Can you work these out from the model? Positions are in its coordinate system, mm. A direction names the side the tool comes from. Give positions to 0.01 mm unless a question says otherwise; leave off trailing zeros. Write each loop counter-clockwise with the first axis right and the second up, starting at its lowest first coordinate (ties: lowest second). Pieces come first, ordered by that corner, then holes.
1. Suppose I cut it at B-B (y = -6.25). Please give me the cut outline in (x, z), and give its area (3 significant figures).
2. Suppose I cut it at A-A (x = 12.5). Please give me the cut outline in (y, z), and give its area (3 significant figures).
3. On a 3-axis mill with a long thin cutter (end or side, diameter ignored), from which of +Z, -Z, +X, -X, +Y, -Y can I reach the whole of each face in a straight line? I mean faces 4 (the flat face through (4.413, -5, -5)), 5 (the flat face through (-5.428, -5, -5)). Say none if no direction works.
4. I'm going to push a flat-ended pin straight in: pin 1 (3 mm diameter, centred on y = -2.5, z = -2.5, fed in from +X). Where does the tip first touch, or does it pass through?
5. Suppose I cut it at C-C (z = -6). Please give me the cut outline in (x, y).
6. If I drill on probe 1 along Z at (x, y) = (4.5, -7); probe 2 along X at (y, z) = (-1.25, -9.5); probe 3 along Y at (x, z) = (4, -4), over which ranges is the centre line in solid material (lowest first)?
7. Thinking about a two-plate mould opening in Z: for faces 1 (the flat face through (9, -5, -15.296)), 2 (the flat face through (2, -10, -5)), 3 (the flat face through (5, -5, 14.704)), which applies, pulls with the +Z half, pulls with the -Z half, needs draft (parallel to the pull), parting line crosses it, or undercut?
```python
from build123d import *

# Parameters (mm, degrees)
F1_DEPTH    = 10
F2_R        = 0.5
F3_R        = 0.5
F4_T1_DEPTH = 11.5


# Not quite as in the source:
# - a fillet or chamfer that OpenCascade refuses, or shapes differently, is made with other operations: its cross-section is extruded or revolved along the edge and cut away or added


with BuildPart() as f1:
    # F0 (on Front) → F1 (new body)
    with BuildSketch(Plane.XZ):
        Polygon((14.5721812431, 14.7042763403), (-5.4278187569, 14.7042763403), (-5.4278187569, -25.2957236597), (14.5721812431, -25.2957236597), (14.5721812431, -15.2957236597), (4.4125382692, -15.2957236597), (4.4125382692, 4.7042763403), (14.5721812431, 4.7042763403), align=None)
    extrude(amount=F1_DEPTH)

    # F2
    f2_edges = [f1.edges().sort_by_distance(p)[0] for p in [
        (14.572181, -10, 9.704276),
        (4.572181, -10, 14.704276),
        (-5.427819, -10, -5.295724),
        (4.572181, -10, -25.295724),
        (14.572181, -10, -20.295724),
        (9.49236, -10, -15.295724),
        (4.412538, -10, -5.295724),
        (9.49236, -10, 4.704276),
    ]]
    fillet(f2_edges, radius=F2_R)

    # F3
    f3_edges = [f1.edges().sort_by_distance(p)[0] for p in [
        (14.572181, 0, 9.704276),
        (4.572181, 0, 14.704276),
        (-5.427819, 0, -5.295724),
        (4.572181, 0, -25.295724),
        (14.572181, 0, -20.295724),
        (9.49236, 0, -15.295724),
        (4.412538, 0, -5.295724),
        (9.49236, 0, 4.704276),
    ]]
    fillet(f3_edges, radius=F3_R)

    # F4: fillet of radius 0.5 on 16 edges, made by hand

    # F4_s2 → F4_t1 (cut)
    with BuildSketch(Plane.XZ.offset(-0.75)):
        with BuildLine():
            ThreePointArc((14.0721812431, -25.2957236597), (14.4257346337, -25.1492770503), (14.5721812431, -24.7957236597))
            Line((14.5721812431, -24.7957236597), (14.5721812431, -25.2957236597))
            Line((14.5721812431, -25.2957236597), (14.0721812431, -25.2957236597))
        make_face()
        with BuildLine():
            ThreePointArc((14.0721812431, -15.2957236597), (14.4257346337, -15.4421702691), (14.5721812431, -15.7957236597))
            Line((14.5721812431, -15.7957236597), (14.5721812431, -15.2957236597))
            Line((14.5721812431, -15.2957236597), (14.0721812431, -15.2957236597))
        make_face()
        with BuildLine():
            ThreePointArc((-5.4278187569, -24.7957236597), (-5.2813721475, -25.1492770503), (-4.9278187569, -25.2957236597))
            Line((-4.9278187569, -25.2957236597), (-5.4278187569, -25.2957236597))
            Line((-5.4278187569, -25.2957236597), (-5.4278187569, -24.7957236597))
        make_face()
        with BuildLine():
            ThreePointArc((14.5721812431, 5.2042763403), (14.4257346337, 4.8507229497), (14.0721812431, 4.7042763403))
            Line((14.0721812431, 4.7042763403), (14.5721812431, 4.7042763403))
            Line((14.5721812431, 4.7042763403), (14.5721812431, 5.2042763403))
        make_face()
        with BuildLine():
            ThreePointArc((14.5721812431, 14.2042763403), (14.4257346337, 14.5578297309), (14.0721812431, 14.7042763403))
            Line((14.0721812431, 14.7042763403), (14.5721812431, 14.7042763403))
            Line((14.5721812431, 14.7042763403), (14.5721812431, 14.2042763403))
        make_face()
        with BuildLine():
            ThreePointArc((-4.9278187569, 14.7042763403), (-5.2813721475, 14.5578297309), (-5.4278187569, 14.2042763403))
            Line((-5.4278187569, 14.2042763403), (-5.4278187569, 14.7042763403))
            Line((-5.4278187569, 14.7042763403), (-4.9278187569, 14.7042763403))
        make_face()
    extrude(amount=F4_T1_DEPTH, mode=Mode.SUBTRACT)


solid = f1.part
```
Checks:
1. outline: (-5.43, -24.8) arc R0.5 ccw to (-4.93, -25.3) - (14.07, -25.3) arc R0.5 ccw to (14.57, -24.8) - (14.57, -15.8) arc R0.5 ccw to (14.07, -15.3) - (4.41, -15.3) - (4.41, 4.7) - (14.07, 4.7) arc R0.5 ccw to (14.57, 5.2) - (14.57, 14.2) arc R0.5 ccw to (14.07, 14.7) - (-4.93, 14.7) arc R0.5 ccw to (-5.43, 14.2) - close
1. area: 596 mm2
2. outline: (-10, -24.8) arc R0.5 ccw to (-9.5, -25.3) - (-0.5, -25.3) arc R0.5 ccw to (0, -24.8) - (0, -15.8) arc R0.5 ccw to (-0.5, -15.3) - (-9.5, -15.3) arc R0.5 ccw to (-10, -15.8) - close; (-10, 5.2) arc R0.5 ccw to (-9.5, 4.7) - (-0.5, 4.7) arc R0.5 ccw to (0, 5.2) - (0, 14.2) arc R0.5 ccw to (-0.5, 14.7) - (-9.5, 14.7) arc R0.5 ccw to (-10, 14.2) - close
2. area: 200 mm2
3. face 4: +X, +Y, -Y
3. face 5: +Z, -Z, -X, +Y, -Y
4. pin 1: stops at x = 4.41
5. outline: (-5.43, -9.5) arc R0.5 ccw to (-4.93, -10) - (3.91, -10) arc R0.5 ccw to (4.41, -9.5) - (4.41, -0.5) arc R0.5 ccw to (3.91, 0) - (-4.93, 0) arc R0.5 ccw to (-5.43, -0.5) - close
6. probe 1: z = -25.3 to -15.3, 4.7 to 14.7
6. probe 2: x = -5.43 to 4.41
6. probe 3: y = -9.99 to -0.01
7. face 1: undercut
7. face 2: needs draft
7. face 3: pulls with the +Z half
